Work out the finished part from the listing and answer in its coordinate system (mm). Face numbers are marked on the shaded views. A direction names the side the tool comes from. Coordinates: 2 decimals unless noted, no trailing zeros. Write each loop counter-clockwise with the first axis right and the second up, starting at its lowest first coordinate (ties: lowest second). Pieces come first, ordered by that corner, then holes. Notation, with made-up numbers: (59.5, 48) -> (82.5, 48) arc R25 cw to (82.5, 72) -> close; hole circle Ø8 at (63, 42). An arc over 180 degrees is marked (long way). Write each question's results on one line, items separated by ' | '. Start each with the question number.
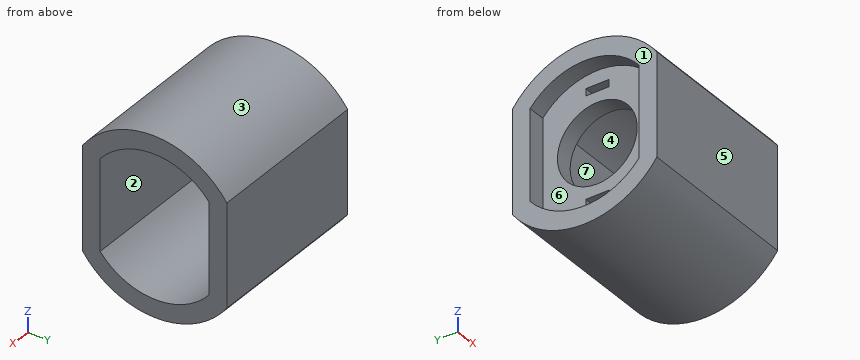
from build123d import *

# Parameters (mm, degrees)
SKETCH_1_W        = 0.8
SKETCH_1_H        = 2.6
SKETCH_1_R        = 4.5
EXTRUDE_1_DEPTH   = 2
EXTRUDE_START     = -4
EXTRUDE_1_2_DEPTH = 19


# Read off the part's stored shape, not the designer's step: 拉伸-薄壁1
with BuildPart() as part:
    # 草图1 → Extrude 1 (new body)
    with BuildSketch(Plane(origin=(0, 0, 0), x_dir=(0, 0, -1), z_dir=(1, 0, 0))):
        with BuildLine():
            ThreePointArc((-5.116395215, 6.15), (-8, 0), (-5.116395215, -6.15))
            Line((-5.116395215, -6.15), (5.116395215, -6.15))
            ThreePointArc((5.116395215, -6.15), (7.243312837, -3.396236025), (8, 0))
            ThreePointArc((8, 0), (7.243312837, 3.396236025), (5.116395215, 6.15))
            Line((5.116395215, 6.15), (-5.116395215, 6.15))
        make_face()
        with Locations((-6.1, 0)):
            Rectangle(SKETCH_1_W, SKETCH_1_H, mode=Mode.SUBTRACT)
        Circle(SKETCH_1_R, mode=Mode.SUBTRACT)
        with Locations((6.1, 0)):
            Rectangle(SKETCH_1_W, SKETCH_1_H, mode=Mode.SUBTRACT)
    extrude(amount=-EXTRUDE_1_DEPTH)

    # Extrude 1 2 outline → Extrude 1 2 (add)
    with BuildSketch(Plane(origin=(0, 0, 0), x_dir=(0, 0, -1), z_dir=(1, 0, 0)).offset(EXTRUDE_START)):
        with BuildLine():
            Line((5.794609564, 8.15), (-5.794609564, 8.15))
            ThreePointArc((-5.794609564, 8.15), (-10, 0), (-5.794609564, -8.15))
            Line((-5.794609564, -8.15), (5.794609564, -8.15))
            ThreePointArc((5.794609564, -8.15), (10, 0), (5.794609564, 8.15))
        make_face()
        with BuildLine():
            ThreePointArc((-5.116395215, -6.15), (-8, 0), (-5.116395215, 6.15))
            Line((-5.116395215, 6.15), (5.116395215, 6.15))
            ThreePointArc((5.116395215, 6.15), (8, 0), (5.116395215, -6.15))
            Line((5.116395215, -6.15), (-5.116395215, -6.15))
        make_face(mode=Mode.SUBTRACT)
    extrude(amount=EXTRUDE_1_2_DEPTH)


solid = part.part
1. Find section D-D on x = 5. Give the vertices of the cut face in (y, z), and give its area (3 significant figures).
2. Find the intervals of material crossed by L1, parallel to Z at x = -1, y = -0.25; L2, parallel to Y at x = -0.6, z = 0; L3, parallel to Y at x = 2.25, z = 2.5, in increasing order.
3. Find section A-A on z = 0. Give the vertices of the cut face in (x, y), and give its area (3 significant figures).
4. Find section B-B on y = 0. Give the vertices of the cut face in (x, z), and give its area (3 significant figures).
5. Given pin 1 Ø3.5 at (y, z) = (-2, -1) entering from +X; pin 2 Ø0.9 at (x, z) = (-1, -6.5) entering from +Y, each flat-ended and moving along its own axis, determine where each tip first touches the part or whether it passes through.
6. Determine the mould class of the marked faces 1, 2, 3 and 4 for opening direction Z: pulls with the +Z half, pulls with the -Z half, needs draft (parallel to the pull), parting line crosses it, or undercut.
7. For the marked faces 5, 6 and 7, determine the directions among +Z, -Z, +X, -X, +Y, -Y from which every point of the face is accessible in a straight line to the end or side of a thin tool.
8. Find section C-C on x = -0.75. Give the vertices of the cut face in (y, z).
Ans:
1) outline: (-8.15, -5.79) arc R10 ccw to (8.15, -5.79) -> (8.15, 5.79) arc R10 ccw to (-8.15, 5.79) -> close; hole (-6.15, -5.12) arc R8 ccw to (6.15, -5.12) -> (6.15, 5.12) arc R8 ccw to (-6.15, 5.12) -> close | area: 110 mm²
2) L1: z = -10 to -6.5, -5.7 to -4.49, 4.49 to 5.7, 6.5 to 10 | L2: y = -8.15 to -4.5, 4.5 to 8.15 | L3: y = -8.15 to -6.15, 6.15 to 8.15
3) outline: (-4, -8.15) -> (15, -8.15) -> (15, -6.15) -> (0, -6.15) -> (0, -4.5) -> (-2, -4.5) -> (-2, -6.15) -> (-4, -6.15) -> close; (-4, 6.15) -> (-2, 6.15) -> (-2, 4.5) -> (0, 4.5) -> (0, 6.15) -> (15, 6.15) -> (15, 8.15) -> (-4, 8.15) -> close | area: 82.6 mm²
4) outline: (-4, -10) -> (15, -10) -> (15, -8) -> (0, -8) -> (0, -6.5) -> (-2, -6.5) -> (-2, -8) -> (-4, -8) -> close; (-4, 8) -> (-2, 8) -> (-2, 6.5) -> (0, 6.5) -> (0, 8) -> (15, 8) -> (15, 10) -> (-4, 10) -> close; (-2, -5.7) -> (0, -5.7) -> (0, -4.5) -> (-2, -4.5) -> close; (-2, 4.5) -> (0, 4.5) -> (0, 5.7) -> (-2, 5.7) -> close | area: 86.8 mm²
5) pin 1: passes through | pin 2: stops at y = 7.96
6) face 1: needs draft | face 2: undercut | face 3: pulls with the +Z half | face 4: undercut
7) face 5: +Z, -Z, +X, -X, -Y | face 6: -X | face 7: +X
8) outline: (-8.15, -5.79) arc R10 ccw to (8.15, -5.79) -> (8.15, 5.79) arc R10 ccw to (-8.15, 5.79) -> close; hole circle Ø9 at (0, 0); hole (-1.3, -6.5) -> (1.3, -6.5) -> (1.3, -5.7) -> (-1.3, -5.7) -> close; hole (-1.3, 5.7) -> (1.3, 5.7) -> (1.3, 6.5) -> (-1.3, 6.5) -> close
